Geometry: final body of the model. Coordinates: model frame, mm. Give positions to 0.01 mm unless a question says otherwise; leave off trailing zeros. One line per item, written item: value.
Autodesk Fusion 360 part; units mm, degrees
sketch "Sketch1" plane through (0, 0, 0) normal (0, 0, 1) x (1, 0, 0)
  circle A0 centre (0, 0) radius 41.275
  circle A1 centre (0, 0) radius 38.735
  circle A2 centre (0, 0) radius 4.445
  dimension "d1" = 82.55
  dimension "d2" = 77.47
  dimension "d5" = 8.89
extrude "Extrude1" add sketch "Sketch1" along normal blind 2.54 makes body 1 at (41.2237, -2.0574, 1.6933) makes body 2 at (4.4229, -0.4426, 0.8467)
sketch "Sketch4" plane through (0, 0, 0) normal (0, 0, 1) x (1, 0, 0)
  line L0 (-1.27, 39.37) -> (1.27, 39.37)
  line L1 (1.27, 39.37) -> (1.27, 1.27)
  line L2 (1.27, 1.27) -> (-1.27, 1.27)
  line L3 (-1.27, 1.27) -> (-1.27, 39.37)
  dimension "d12" = 2.54
  dimension "d13" = 1.27
  dimension "d14" = 38.1
  dimension "d15" = 1.27
extrude "Extrude3" add sketch "Sketch4" along normal blind 2.54 separate body makes body 3
pattern_circular "C-Pattern1" count 4 over 360 about axis through (0, 0, 1.75) along (0, 0, 1) of bodies 3 makes body 4 at (-26.67, 1.27, 0.8467) makes body 5 at (-1.27, -26.67, 0.8467) makes body 6 at (26.67, -1.27, 0.8467)
combine "Combine1" operation add target body 3 tool bodies 1 2 6 5 4
fillet "Fillet1" radius 2.54 8 edges at (4.2597, 1.27, 1.27) (1.27, 4.2597, 1.27) (-1.27, 4.2597, 1.27) (-4.2597, 1.27, 1.27) (-4.2597, -1.27, 1.27) (-1.27, -4.2597, 1.27) (1.27, -4.2597, 1.27) (4.2597, -1.27, 1.27) on bodies 3
fillet "Fillet2" radius 2.54 8 edges at (1.27, -38.7142, 1.27) (-1.27, -38.7142, 1.27) (-38.7142, -1.27, 1.27) (-38.7142, 1.27, 1.27) (-1.27, 38.7142, 1.27) (1.27, 38.7142, 1.27) (38.7142, 1.27, 1.27) (38.7142, -1.27, 1.27) on bodies 3
sketch "Sketch5" plane through (0, 0, 0) normal (1, 0, 0) x (0, 1, 0)
  line L0 (-41.275, 2.54) -> (-40.8209, 2.159)
  line L1 (-40.8209, 2.159) -> (-40.8209, 0.381)
  line L2 (-40.8209, 0.381) -> (-41.275, 0)
  line L3 (-41.275, 2.54) -> (-41.275, 0)
  dimension "d24" = 1.778
  dimension "d25" = 2.54
  dimension "d26" = 130
  dimension "d27" = 130
  dimension "d28" = 41.275
revolve "Revolve1" cut sketch "Sketch5" angle 360 about axis through (0, 0, 1.75) along (0, 0, 1) bodies 3
hole "Hole1" at (0, 0, 2.54) direction (0, 0, -1) diameter 1.6256 depth 6.35 tip angle 118 bodies 3
sketch "Sketch6" plane through (0, 0, 2.54) normal (0, 0, 1) x (-1, 0, 0)
  circle A0 centre (0, 0) radius 0.8115
  arc A1 (4.0774, -38.5198) -> (38.5198, -4.0774) centre (0, 0) ccw
  arc A2 (1.27, -35.9939) -> (4.0774, -38.5198) centre (3.81, -35.9939) ccw
  line L0 (1.27, -35.9939) -> (1.27, -5.8544)
  arc A3 (2.4245, -3.7255) -> (1.27, -5.8544) centre (3.81, -5.8544) ccw
  arc A4 (2.4245, -3.7255) -> (3.7255, -2.4245) centre (0, 0) ccw
  arc A5 (5.8544, -1.27) -> (3.7255, -2.4245) centre (5.8544, -3.81) ccw
  line L1 (5.8544, -1.27) -> (35.9939, -1.27)
  arc A6 (38.5198, -4.0774) -> (35.9939, -1.27) centre (35.9939, -3.81) ccw
  line L2 (-35.9939, -1.27) -> (-5.8544, -1.27)
  arc A7 (-3.7255, -2.4245) -> (-5.8544, -1.27) centre (-5.8544, -3.81) ccw
  arc A8 (-3.7255, -2.4245) -> (-2.4245, -3.7255) centre (0, 0) ccw
  arc A9 (-1.27, -5.8544) -> (-2.4245, -3.7255) centre (-3.81, -5.8544) ccw
  line L3 (-1.27, -5.8544) -> (-1.27, -35.9939)
  arc A10 (-4.0774, -38.5198) -> (-1.27, -35.9939) centre (-3.81, -35.9939) ccw
  arc A11 (-38.5198, -4.0774) -> (-4.0774, -38.5198) centre (0, 0) ccw
  arc A12 (-35.9939, -1.27) -> (-38.5198, -4.0774) centre (-35.9939, -3.81) ccw
  circle A13 centre (0, 0) radius 41.275
  line L4 (-1.27, 35.9939) -> (-1.27, 5.8544)
  arc A14 (-2.4245, 3.7255) -> (-1.27, 5.8544) centre (-3.81, 5.8544) ccw
  arc A15 (-2.4245, 3.7255) -> (-3.7255, 2.4245) centre (0, 0) ccw
  arc A16 (-5.8544, 1.27) -> (-3.7255, 2.4245) centre (-5.8544, 3.81) ccw
  line L5 (-5.8544, 1.27) -> (-35.9939, 1.27)
  arc A17 (-38.5198, 4.0774) -> (-35.9939, 1.27) centre (-35.9939, 3.81) ccw
  arc A18 (-4.0774, 38.5198) -> (-38.5198, 4.0774) centre (0, 0) ccw
  arc A19 (-1.27, 35.9939) -> (-4.0774, 38.5198) centre (-3.81, 35.9939) ccw
  line L6 (35.9939, 1.27) -> (5.8544, 1.27)
  arc A20 (3.7255, 2.4245) -> (5.8544, 1.27) centre (5.8544, 3.81) ccw
  arc A21 (3.7255, 2.4245) -> (2.4245, 3.7255) centre (0, 0) ccw
  arc A22 (1.27, 5.8544) -> (2.4245, 3.7255) centre (3.81, 5.8544) ccw
  line L7 (1.27, 5.8544) -> (1.27, 35.9939)
  arc A23 (4.0774, 38.5198) -> (1.27, 35.9939) centre (3.81, 35.9939) ccw
  arc A24 (38.5198, 4.0774) -> (4.0774, 38.5198) centre (0, 0) ccw
  arc A25 (35.9939, 1.27) -> (38.5198, 4.0774) centre (35.9939, 3.81) ccw
fillet "Fillet3" radius 1.27 2 edges at (-38.0585, -14.7615, 2.159) (-38.0585, -14.7615, 0.381) on bodies 3
sketch "Sketch8" plane through (0, 0, 0) normal (0, 0, -1) x (1, 0, 0)
  circle A0 centre (0, 0) radius 0.8115
  arc A1 (-1.27, 35.9939) -> (-4.0774, 38.5198) centre (-3.81, 35.9939) ccw
  line L0 (-1.27, 35.9939) -> (-1.27, 5.8544)
  arc A2 (-2.4245, 3.7255) -> (-1.27, 5.8544) centre (-3.81, 5.8544) ccw
  arc A3 (-2.4245, 3.7255) -> (-3.7255, 2.4245) centre (0, 0) ccw
  arc A4 (-5.8544, 1.27) -> (-3.7255, 2.4245) centre (-5.8544, 3.81) ccw
  line L1 (-5.8544, 1.27) -> (-35.9939, 1.27)
  arc A5 (-38.5198, 4.0774) -> (-35.9939, 1.27) centre (-35.9939, 3.81) ccw
  arc A6 (-4.0774, 38.5198) -> (-38.5198, 4.0774) centre (0, 0) ccw
  line L2 (-35.9939, -1.27) -> (-5.8544, -1.27)
  arc A7 (-3.7255, -2.4245) -> (-5.8544, -1.27) centre (-5.8544, -3.81) ccw
  arc A8 (-3.7255, -2.4245) -> (-2.4245, -3.7255) centre (0, 0) ccw
  arc A9 (-1.27, -5.8544) -> (-2.4245, -3.7255) centre (-3.81, -5.8544) ccw
  line L3 (-1.27, -5.8544) -> (-1.27, -35.9939)
  arc A10 (-4.0774, -38.5198) -> (-1.27, -35.9939) centre (-3.81, -35.9939) ccw
  arc A11 (-38.5198, -4.0774) -> (-4.0774, -38.5198) centre (0, 0) ccw
  arc A12 (-35.9939, -1.27) -> (-38.5198, -4.0774) centre (-35.9939, -3.81) ccw
  arc A13 (35.9939, 1.27) -> (38.5198, 4.0774) centre (35.9939, 3.81) ccw
  line L4 (35.9939, 1.27) -> (5.8544, 1.27)
  arc A14 (3.7255, 2.4245) -> (5.8544, 1.27) centre (5.8544, 3.81) ccw
  arc A15 (3.7255, 2.4245) -> (2.4245, 3.7255) centre (0, 0) ccw
  arc A16 (1.27, 5.8544) -> (2.4245, 3.7255) centre (3.81, 5.8544) ccw
  line L5 (1.27, 5.8544) -> (1.27, 35.9939)
  arc A17 (4.0774, 38.5198) -> (1.27, 35.9939) centre (3.81, 35.9939) ccw
  arc A18 (38.5198, 4.0774) -> (4.0774, 38.5198) centre (0, 0) ccw
  line L6 (1.27, -35.9939) -> (1.27, -5.8544)
  arc A19 (2.4245, -3.7255) -> (1.27, -5.8544) centre (3.81, -5.8544) ccw
  arc A20 (2.4245, -3.7255) -> (3.7255, -2.4245) centre (0, 0) ccw
  arc A21 (5.8544, -1.27) -> (3.7255, -2.4245) centre (5.8544, -3.81) ccw
  line L7 (5.8544, -1.27) -> (35.9939, -1.27)
  arc A22 (38.5198, -4.0774) -> (35.9939, -1.27) centre (35.9939, -3.81) ccw
  arc A23 (4.0774, -38.5198) -> (38.5198, -4.0774) centre (0, 0) ccw
  arc A24 (1.27, -35.9939) -> (4.0774, -38.5198) centre (3.81, -35.9939) ccw
  circle A25 centre (0, 0) radius 41.275
  line L8 (-2.0319, 1.778) -> (2.0319, 1.778)
  line L9 (-2.0319, -1.778) -> (2.0319, -1.778)
  arc A26 (-2.0319, 1.778) -> (-2.0319, -1.778) centre (0, 0) ccw
  arc A27 (2.0319, -1.778) -> (2.0319, 1.778) centre (0, 0) ccw
  dimension "d42" = 5.4
  dimension "d43" = 3.556
extrude "Extrude4" cut sketch "Sketch8" against normal blind 1.27 contours L8 L9 A26 A27 bodies 3
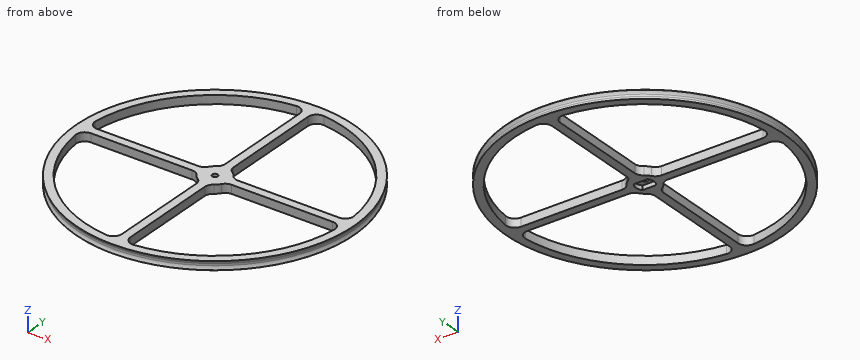
1) First-contact query: pin 1 (1.3 mm diameter, centred on x = 25.5, z = 1.5, fed in from -Y); pin 2 (0.8 mm diameter, centred on x = 16.5, z = 1.5, fed in from +Y); pin 3 (6 mm diameter, centred on x = -29, y = -20.5, fed in from -Z); pin 4 (1.3 mm diameter, centred on y = 28, z = 1.5, fed in from -X). Flat tips, straight axial feed; report the tip coordinate or a pass-through.
Answers below:
pin 1: y = -32.39
pin 2: y = 37.51
pin 3: through
pin 4: x = -30.3
2) Section A-A, the plane x = 21.5. Count the separate pieces of the cut face and the enclosed holes in it, then the cut area to 3 significant figures.
Answers below:
separate pieces: 3
enclosed holes: 0
area: 19.7 mm^2
3) Material intervals for line 1 along X through (y, z) = (0, 1.65); line 2 along X through (y, z) = (35, 0.6); line 3 along Y through (x, z) = (9.5, 1.75), sorted ascending.
Answers below:
line 1: -40.82 to -0.81, 0.81 to 40.82
line 2: -21.12 to -16.6, -1.27 to 1.27, 16.6 to 21.12
line 3: -39.71 to -37.55, -1.27 to 1.27, 37.55 to 39.71
